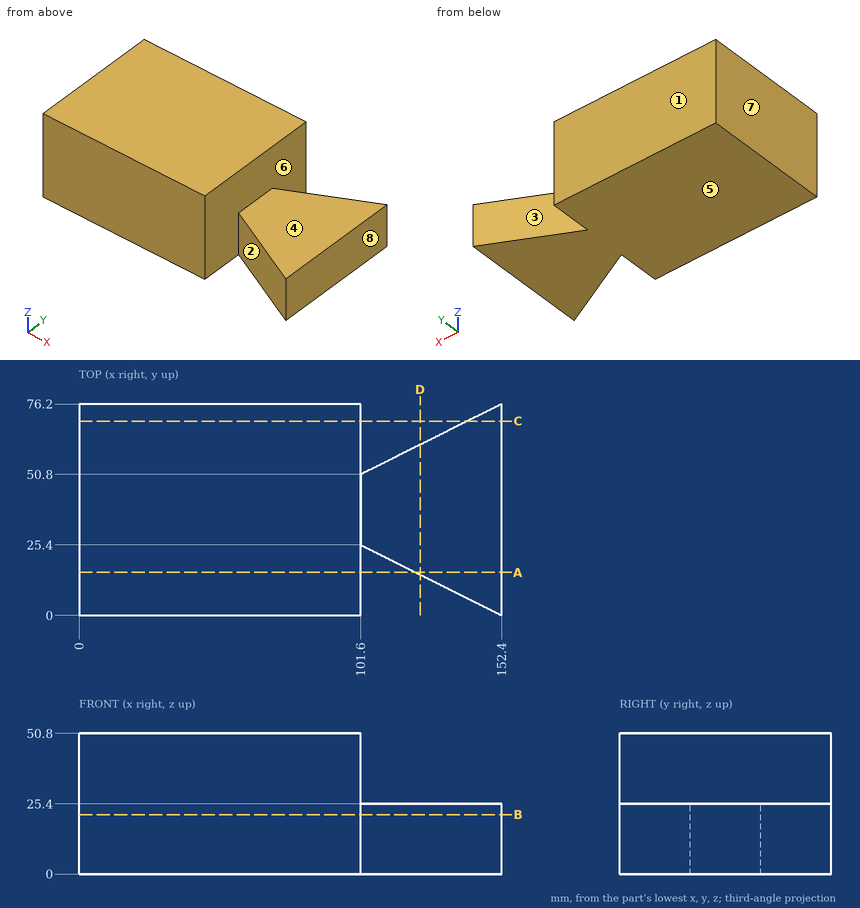
Could you check a few things on this drawing? It's one solid part, dimensions in mm from its lowest x, y, z. A direction names the side the tool comes from. Coordinates: 2 decimals unless noted, no trailing zeros. Order: outer loops, then holes, each group sorted by start corner. A loop starts at its lowest first (then second) coordinate and runs counter-clockwise, first axis right, second up. Notation, with made-up numbers: (-39, 69.5) -> (16, 69.5) arc R14 cw to (16, 83.5) -> close; hole circle Ø8 at (76, -27.75). An arc over 180 degrees is marked (long way). One line per item, written item: value. Start each with the question number.
1) Which directions (+Z, -Z, +X, -X, +Y, -Y) give clear straight access to the entire face, cutting with the end or side of a thin tool? Please do the marked faces 1, 2, 3 and 4.
2) Imagine slicing it at B-B on z = 21.5. List the corners of the cut face in (x, y) for me, plus the area to 3 significant figures.
3) Imagine slicing it at A-A on y = 15.5. List the corners of the cut face in (x, z) for me, plus the area to 3 significant figures.
4) We'd pull the mould along X, two halves only. Please class the marked faces 5, 6, 7 and 8: +X half, -X half, draft (parallel to the pull), parting line (faces both ways), or undercut.
5) Imagine slicing it at D-D on x = 123. List the corners of the cut face in (y, z) for me.
6) Imagine slicing it at C-C on y = 70. List the corners of the cut face in (x, z) for me, plus the area to 3 significant figures.
7) If I drill on L1, parallel to X at y = 50, z = 36; L2, parallel to Z at x = 125, y = 37; L3, parallel to X at y = 16.5, z = 20, over which ranges is the centre line in solid material (lowest first)? Write a range as [from, to].
Answer list:
1. face 1: +Z, -Z, +X, -X, +Y
1. face 2: +Z, -Z, -Y
1. face 3: +Z, -Z, +Y
1. face 4: +Z, +X, +Y, -Y
2. outline: (0, 0) -> (101.6, 0) -> (101.6, 25.4) -> (152.4, 0) -> (152.4, 76.2) -> (101.6, 50.8) -> (101.6, 76.2) -> (0, 76.2) -> close
2. area: 10,300 mm2
3. outline: (0, 0) -> (101.6, 0) -> (101.6, 50.8) -> (0, 50.8) -> close; (121.4, 0) -> (152.4, 0) -> (152.4, 25.4) -> (121.4, 25.4) -> close
3. area: 5,950 mm2
4. face 5: draft
4. face 6: undercut
4. face 7: -X half
4. face 8: +X half
5. outline: (14.7, 0) -> (61.5, 0) -> (61.5, 25.4) -> (14.7, 25.4) -> close
6. outline: (0, 0) -> (101.6, 0) -> (101.6, 50.8) -> (0, 50.8) -> close; (140, 0) -> (152.4, 0) -> (152.4, 25.4) -> (140, 25.4) -> close
6. area: 5,480 mm2
7. L1: x = [0, 101.6]
7. L2: z = [0, 25.4]
7. L3: x = [0, 101.6], [119.4, 152.4]
